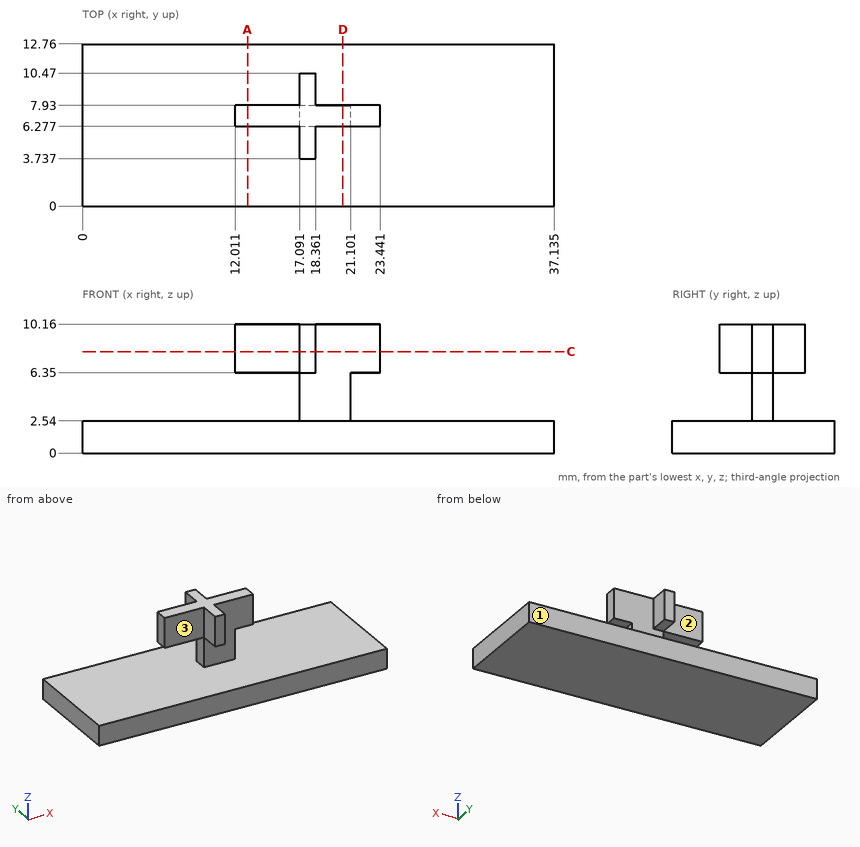
Design review of the part shown in the three views and the two pictorial views. Dimensions are in mm from the part's minimum x, y and z. A direction names the side the tool comes from. Give positions to 0.01 mm unless a question says otherwise; leave off trailing zeros. Loops run counter-clockwise (first coordinate to the right, second up) from the corner with the lowest first, then second, coordinate; pieces in that order, holes last. Notation, with made-up numbers: M 10,66.25 L 16,66.25 A20 cw 16,103.25 Z; hole C 26.25,5.5 d2. An arc over 180 degrees is marked long. Answer as a JSON object with one key per item and string values. Group by question number.
Q1. Add section C-C on z = 8. Give the boundary of the cut face in (x, y).
Q2. Add section A-A on x = 13. Give the boundary of the cut face in (y, z), and give its area (3 significant figures).
Q3. Tool access review of the marked faces 1, 2 and 3: name each direction out of +Z, -Z, +X, -X, +Y, -Y from which nothing blocks a thin tool from reaching the whole face with its end or side.
Q4. Insertion check: P1, Ø0.5, axis at y = 7.5, z = 7.5, coming from the +X side; P2, Ø4, axis at x = 15, z = 9, coming from the -Y side; P3, Ø0.6, axis at x = 17.5, z = 8, coming from the +Y side. Each pin has a flat end and moves straight along its axis. Give the tip position at first contact, or say it passes through.
Q5. For probe 1 along Z at (x, y) = (18.5, 1); probe 2 along X at (y, z) = (7, 9.5); probe 3 along X at (y, z) = (5.25, 8.25), list the stretches that pass through material, from the lowest coordinate up. Write a range as [from, to].
Q6. Add section D-D on x = 20.5. Give the boundary of the cut face in (y, z), and give its area (3 significant figures).
Checked values:
{
 "1": {"outline": "M 12.01,6.28 L 17.09,6.28 L 17.09,3.74 L 18.36,3.74 L 18.36,6.28 L 23.44,6.28 L 23.44,7.93 L 18.36,7.93 L 18.36,10.47 L 17.09,10.47 L 17.09,7.93 L 12.01,7.93 Z"},
 "2": {"outline": "M 0,0 L 12.76,0 L 12.76,2.54 L 0,2.54 Z; M 6.28,6.35 L 7.93,6.35 L 7.93,10.16 L 6.28,10.16 Z", "area": "38.7 mm²"},
 "3": {"face 1": "+Z, -Z, +X, -X, +Y", "face 2": "+Z, -X, +Y", "face 3": "+Z, -X, -Y"},
 "4": {"P1": "x = 23.44", "P2": "y = 6.28", "P3": "y = 10.47"},
 "5": {"probe 1": "[0, 2.54]", "probe 2": "[12.01, 23.44]", "probe 3": "[17.09, 18.36]"},
 "6": {"outline": "M 0,0 L 12.76,0 L 12.76,2.54 L 7.93,2.54 L 7.93,10.16 L 6.28,10.16 L 6.28,2.54 L 0,2.54 Z", "area": "45.0 mm²"}
}
